from build123d import *

# Parameters (mm, degrees)
F0_R        = 12
F1_DEPTH    = 12
F3_R        = 7.5
F3_W        = 5.5
F3_H        = 5.5
F4_DEPTH    = 1
F4_FACE_R   = 7.5
F1_FACE_R   = 12
F6_DEPTH    = 25
F7_DEPTH    = 12
F8_W        = 8
F8_H        = 8
F8_R        = 1.5
F9_DEPTH    = 20
F9_FACE_W   = 14.6
F9_FACE_H   = 8
F10_DEPTH   = 8
F9_FACE_W_2 = 5.5
F9_FACE_H_2 = 5.5
F11_DEPTH   = 25
F12_DEPTH   = 12.5


with BuildPart() as f1:
    # F0 (on Top) → F1 (new body)
    with BuildSketch(Plane.XY):
        Circle(F0_R)
        Polygon((-7.3, -4.214657), (-7.3, 4.214657), (0, 8.429314), (7.3, 4.214657), (7.3, -4.214657), (0, -8.429314), align=None, mode=Mode.SUBTRACT)
        Polygon((0, 8.429314), (-7.3, 4.214657), (-7.3, -4.214657), (0, -8.429314), (7.3, -4.214657), (7.3, 4.214657), align=None)
    extrude(amount=F1_DEPTH)



with BuildPart() as f4:
    # F3 (on offset) → F4 (new body)
    with BuildSketch(Plane.XY.offset(37)):
        Circle(F3_R)
        Rectangle(F3_W, F3_H, mode=Mode.SUBTRACT)
        Rectangle(F3_W, F3_H)
    extrude(amount=-F4_DEPTH)


with BuildPart() as f1_1:
    add(f1.part)

    add(f4.part)  # F5 merges F4
    # F4_face (on face) → F5 section 0
    with BuildSketch(Plane(origin=(0, 0, 36), x_dir=(1, 0, 0), z_dir=(0, 0, -1))):
        Circle(F4_FACE_R)
    # F1_face (on face) → F5 section 1
    with BuildSketch(Plane.XY.offset(12)):
        Circle(F1_FACE_R)
    loft()

    # F3 (on offset) → F6 (cut)
    with BuildSketch(Plane.XY.offset(37)):
        Rectangle(F3_W, F3_H)
    extrude(amount=-F6_DEPTH, mode=Mode.SUBTRACT)

    # F0 (on Top) → F7 (cut)
    with BuildSketch(Plane.XY):
        Polygon((0, 8.429314), (-7.3, 4.214657), (-7.3, -4.214657), (0, -8.429314), (7.3, -4.214657), (7.3, 4.214657), align=None)
    extrude(amount=F7_DEPTH, mode=Mode.SUBTRACT)

    # F8 (on Right) → F9 (join, symmetric)
    with BuildSketch(Plane.YZ):
        with Locations((0, 22)):
            Rectangle(F8_W, F8_H)
        with Locations((0, 22)):
            Circle(F8_R, mode=Mode.SUBTRACT)
        with Locations((0, 6)):
            Rectangle(F8_W, F8_H)
        with Locations((0, 6)):
            Circle(F8_R, mode=Mode.SUBTRACT)
    extrude(amount=F9_DEPTH, both=True)

    # F9_face (on face) → F10 (cut)
    with BuildSketch(Plane(origin=(0, 0, 2), x_dir=(1, 0, 0), z_dir=(0, 0, -1))):
        Rectangle(F9_FACE_W, F9_FACE_H)
    extrude(amount=-F10_DEPTH, mode=Mode.SUBTRACT)

    # F9_face (on face) → F11 (cut)
    with BuildSketch(Plane(origin=(0, 0, 2), x_dir=(1, 0, 0), z_dir=(0, 0, -1))):
        Rectangle(F9_FACE_W_2, F9_FACE_H_2)
    extrude(amount=-F11_DEPTH, mode=Mode.SUBTRACT)

    # F8 (on Right) → F12 (cut, symmetric)
    with BuildSketch(Plane.YZ):
        with Locations((0, 22)):
            Circle(F8_R)
        with Locations((0, 6)):
            Circle(F8_R)
    extrude(amount=F12_DEPTH, both=True, mode=Mode.SUBTRACT)


solid = f1_1.part
Work out the finished part from the listing and answer in its coordinate system (mm). A direction names the side the tool comes from. Give positions to 0.01 mm unless a question says otherwise; leave off trailing zeros. Loops run counter-clockwise (first coordinate to the right, second up) from the corner with the lowest first, then second, coordinate; pieces in that order, holes last. Notation, with made-up numbers: (18, 36.5) - (24, 36.5) arc R14 ccw to (24, 47.5) - close; hole circle Ø7 at (7.25, 22). An arc over 180 degrees is marked (long way). Answer in a Markdown table with one row per item. Add a question column.
Q1. Consider line 1 along Z through (x, y) = (-17, 0); line 2 along Z through (x, y) = (-9.55, 0); line 3 along Z through (x, y) = (-6.5, 0). Determine where each line is inside the solid, lowest interval first.
Q2. The part is cut by section A-A (x = -13.5). Determine the outline of the cut face in (y, z).
Q3. A tool of negligible diameter and unlimited length cuts with its end or side. For faces 4 (the cylindrical face through (-7.493, 0.33, 36.507)), 5 (the flat face through (-16, 4, 6)), 6 (the flat face through (3.6, -6.35, 5.92)), 7 (the flat face through (-14, 4, 22)), 8 (the flat face through (0, -2.75, 25)), from which of +Z, -Z, +X, -X, +Y, -Y can it reach the whole face along a straight path? Write none if from no direction.
Q4. The part is cut by section C-C (z = 32). Determine the outline of the cut face in (x, y).
Q5. Each of these flat-tipped pins is pushed along its axis until it touches: P1, Ø7.5, axis at x = 2.5, y = 1.5, coming from the -Z side; P2, Ø6.5, axis at x = 15, z = 6.5, coming from the +Y side; P3, Ø6.5, axis at x = -13.5, y = -0.5, coming from the +Z side; P4, Ø1.8, axis at y = 0, z = 22, coming from the +X side. Where does it stop, or does it pass through?
Q6. The part is cut by section D-D (y = 0). State how many separate pieces and enclosed holes the cut face has, and give its area (3 significant figures).
Q7. The part is cut by section B-B (z = 6). Determine the outline of the cut face in (x, y).
Q8. Determine the mould class of faces 1 (the flat face through (5, 6, 0)), 2 (the flat face through (-2.75, 0, 25)), 3 (the flat face through (-16, -4, 6)) for opening direction Y: released by +Y, released by -Y, zero draft, split by the parting line, or undercut.
Solution:
| question | item | result |
|---|---|---|
| 1 | line 1 | z = 2 to 4.5, 7.5 to 10, 18 to 20.5, 23.5 to 26 |
| 1 | line 2 | z = 0 to 4.5, 7.5 to 20.5, 23.5 to 26 |
| 1 | line 3 | z = 12 to 20.5, 23.5 to 37 |
| 2 | outline | (-4, 2) - (4, 2) - (4, 10) - (-4, 10) - close; (-4, 18) - (4, 18) - (4, 26) - (-4, 26) - close; hole circle Ø3 at (0, 6); hole circle Ø3 at (0, 22) |
| 3 | face 4 | +Z |
| 3 | face 5 | +Z, -Z, -X, +Y |
| 3 | face 6 | -Z |
| 3 | face 7 | +Z, -X, +Y |
| 3 | face 8 | +Z, -Z |
| 4 | outline | circle Ø16.5 at (0, 0); hole (-2.75, -2.75) - (2.75, -2.75) - (2.75, 2.75) - (-2.75, 2.75) - close |
| 5 | P1 | stops at z = 12 |
| 5 | P2 | stops at y = 4 |
| 5 | P3 | stops at z = 26 |
| 5 | P4 | passes through |
| 6 | separate pieces | 6 |
| 6 | enclosed holes | 0 |
| 6 | area | 565 mm² |
| 7 | outline | (-20, -4) - (-11.31, -4) arc R12 ccw to (11.31, -4) - (20, -4) - (20, -1.5) - (7.3, -1.5) - (7.3, -4.21) - (0, -8.43) - (-7.3, -4.21) - (-7.3, -1.5) - (-20, -1.5) - close; (-20, 1.5) - (-7.3, 1.5) - (-7.3, 4.21) - (0, 8.43) - (7.3, 4.21) - (7.3, 1.5) - (20, 1.5) - (20, 4) - (11.31, 4) arc R12 ccw to (-11.31, 4) - (-20, 4) - close |
| 8 | face 1 | zero draft |
| 8 | face 2 | undercut |
| 8 | face 3 | released by -Y |
